Can you work these out from the model? Positions are in its coordinate system, mm. A direction names the side the tool comes from. Coordinates: 2 decimals unless noted, no trailing zeros. Order: outer loops, then holes, each group sorted by start corner. A loop starts at its lowest first (then second) coordinate and runs counter-clockwise, first axis right, second up.
Autodesk Inventor part; units mm, degrees
ref_plane "YZ Plane" through (0, 0, 0) normal (1, 0, 0) x (0, 1, 0)
ref_plane "XZ Plane" through (0, 0, 0) normal (0, 1, 0) x (-1, 0, 0)
ref_plane "XY Plane" through (0, 0, 0) normal (0, 0, 1) x (1, 0, 0)
sketch "Sketch1" plane through (0, 0, 0) normal (0, 0, 1) x (1, 0, 0)
  line L0 (0, 0) -> (31.75, 0)
  line L1 (31.75, 0) -> (31.75, 42.935)
  line L2 (31.75, 42.935) -> (0, 42.935)
  line L3 (0, 42.935) -> (0, 0)
  dimension "d0" = 31.75
extrude "Extrusion1" add sketch "Sketch1" along normal blind 3.175
sketch "Sketch2" plane through (0, 0, 0) normal (-1, 0, 0) x (0, 0, 1)
  line L0 (-5.0008, 44.6006) -> (-1.6553, 42.6148)
  arc A0 (0, 40.2857) -> (-1.6553, 42.6148) centre (-3.4548, 39.5831) ccw
  line L1 (-5.0008, 44.6006) -> (-3.3281, 47.2993)
  line L2 (3.175, 0) -> (3.175, 42.935)
  line L3 (-3.3281, 47.2993) -> (3.175, 42.935)
  line L4 (0, 0) -> (0, 42.935)
  line L5 (0, 40.2857) -> (0, 42.935)
  line L6 (0, 42.935) -> (3.175, 42.935)
  dimension "d3" = 3.175
extrude "Extrusion2" add sketch "Sketch2" against normal blind 31.75
fillet "Fillet1" radius 6.35 1 edges at (15.875, 42.935, 3.175)
properties part number "slide plate"
1. Imagine slicing it at B-B on y = 4.5. Please give me the cut outline in (x, z) (3 decimals).
Completed:
outline: (0, 0) - (31.75, 0) - (31.75, 3.175) - (0, 3.175) - close
2. Please list where these lines run through material, in increasing order: probe 1 along Z at (x, y) = (8.5, 17) (3 decimals); probe 2 along Z at (x, y) = (18, 40.5); probe 3 along Y at (x, z) = (23, -2).
Completed:
probe 1: z = 0 to 3.175
probe 2: z = -0.05 to 3.1
probe 3: y = 42.82 to 46.41
3. I'm going to push flat-ended pins straight in: pin 1 (6 mm diameter, centred on x = 27.5, y = 32.5, fed in from -Z); pin 2 (4 mm diameter, centred on x = 12.5, z = 1.5, fed in from +Y); pin 3 (2 mm diameter, centred on y = 8, z = -0.5, fed in from +X). Where does each tip first touch, or does it pass through?
Completed:
pin 1: stops at z = 0
pin 2: stops at y = 45.4
pin 3: stops at x = 31.75
4. Imagine slicing it at A-A on x = 7.5. Please give me the cut outline in (y, z) (3 decimals).
Completed:
outline: (0, 0) - (40.286, 0) arc R3.526 cw to (42.615, -1.655) - (44.601, -5.001) - (47.299, -3.328) - (44.822, 0.364) arc R6.35 ccw to (39.549, 3.175) - (0, 3.175) - close
5. On a 3-axis mill with a long thin cutter (end or side, diameter ignored), from which of +Z, -Z, +X, -X, +Y, -Y can I reach the whole of each face in a straight line? I mean faces 1 (the flat face through (16, 20, 0)), 2 (the flat face through (16, 0, 2)). Say none if no direction works.
Completed:
face 1: -Z, +X, -X, -Y
face 2: +Z, -Z, +X, -X, -Y
6. Imagine slicing it at C-C on z = 1.75. Please give me the cut outline in (x, y).
Completed:
outline: (0, 0) - (31.75, 0) - (31.75, 43.56) - (0, 43.56) - close
